Could you check a few things on this model? Use its own coordinates, in mm. Face numbers are marked on the shaded views. A direction names the side the tool comes from. Give positions to 0.01 mm unless a question says otherwise; leave off trailing zeros. Loops run counter-clockwise (first coordinate to the right, second up) from the corner with the lowest first, then second, coordinate; pieces in that order, holes last. Notation, with made-up numbers: (-20.5, -28) -> (-16.5, -28) arc R36 ccw to (-16.5, 7) -> close; hole circle Ø5 at (80, -9). An arc over 180 degrees is marked (long way). Put each result on its own line as item: value.
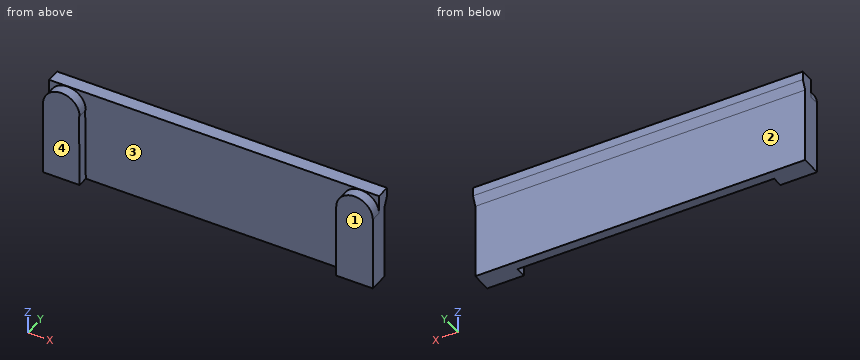
```python
from build123d import *

# Parameters (mm, degrees)
CROQUIS1_W              = 747.21
CROQUIS1_H              = 211.28
SALIENTE_EXTRUIR1_DEPTH = 22
SALIENTE_EXTRUIR6_DEPTH = 39


with BuildPart() as part:
    # Croquis1 → Saliente-Extruir1 (new body)
    with BuildSketch(Plane(origin=(0, 0, 0), x_dir=(1, 0, 0), z_dir=(0, 1, 0))):
        with Locations((318.109210015, -105.64)):
            Rectangle(CROQUIS1_W, CROQUIS1_H)
    extrude(amount=SALIENTE_EXTRUIR1_DEPTH)

    # Croquis2 → Recubrir1 section 0
    with BuildSketch(Plane(origin=(0, 22, 0), x_dir=(1, 0, 0), z_dir=(0, 1, 0))):
        with BuildLine():
            Line((-55.495789985, -171.71895061), (-55.495789985, -211.28))
            Line((-55.495789985, -211.28), (691.714210015, -211.28))
            Line((691.714210015, -211.28), (691.714210015, -171.71895061))
            Line((691.714210015, -171.71895061), (-55.495789985, -171.71895061))
        make_face()
    # Croquis3 → Recubrir1 section 1
    with BuildSketch(Plane(origin=(0, 31, 0), x_dir=(1, 0, 0), z_dir=(0, 1, 0))):
        with BuildLine():
            Line((-55.495789985, -211.28), (-55.495789985, -191.499475305))
            Line((-55.495789985, -191.499475305), (691.714210015, -191.499475305))
            Line((691.714210015, -191.499475305), (691.714210015, -211.28))
            Line((691.714210015, -211.28), (-55.495789985, -211.28))
        make_face()
    loft()

    # Croquis4 → Saliente-Extruir6 (add)
    with BuildSketch(Plane(origin=(0, -24, 0), x_dir=(-1, 0, 0), z_dir=(0, -1, 0))):
        with BuildLine():
            Line((-691.714210015, 0), (-608.79118576, 0))
            Line((-608.79118576, 0), (-608.79118576, -169.061248366))
            ThreePointArc((-608.79118576, -169.061248366), (-650.252697887, -210.522760493), (-691.714210015, -169.061248366))
            Line((-691.714210015, -169.061248366), (-691.714210015, 0))
        make_face()
        with BuildLine():
            Line((55.495789985, 0), (55.495789985, -169.06124837))
            ThreePointArc((55.495789985, -169.06124837), (14.034277855, -210.5227605), (-27.427234275, -169.06124837))
            Line((-27.427234275, -169.06124837), (-26.075334487, -168.034902921))
            Line((-26.075334487, -168.034902921), (-27.427234275, 0))
            Line((-27.427234275, 0), (55.495789985, 0))
        make_face()
    extrude(amount=-SALIENTE_EXTRUIR6_DEPTH)


solid = part.part
```
1. If we section it at A-A (y = -16.5): List the corners of the cut face in (x, z) for me, then the cut area to 3 significant figures.
Recorded:
outline: (-55.5, 0) -> (27.43, 0) -> (26.08, 168.03) -> (27.43, 169.06) arc R41.46 ccw to (-55.5, 169.06) -> close; (608.79, 0) -> (691.71, 0) -> (691.71, 169.06) arc R41.46 ccw to (608.79, 169.06) -> close
area: 33,300 mm^2
2. I'm going to push flat-ended pins straight in: pin 1 (3 mm diameter, centred on x = 213.5, z = 108.5, fed in from -Y); pin 2 (1.5 mm diameter, centred on x = 554, z = 178.5, fed in from +Y); pin 3 (3 mm diameter, centred on x = 581.5, z = 91.5, fed in from +Y). Where does each tip first touch, or does it pass through?
Recorded:
pin 1: stops at y = 0
pin 2: stops at y = 25.43
pin 3: stops at y = 22
3. If we section it at C-C (z = 97): List the corners of the cut face in (x, y) for me, then the cut area to 3 significant figures.
Recorded:
outline: (-55.5, -24) -> (26.65, -24) -> (26.65, 0) -> (608.79, 0) -> (608.79, -24) -> (691.71, -24) -> (691.71, 22) -> (-55.5, 22) -> close
area: 20,400 mm^2
4. Thinking about a two-plate mould opening in X: for the marked faces 3 and 4, which applies, pulls with the +X half, pulls with the -X half, needs draft (parallel to the pull), parting line crosses it, or undercut?
Recorded:
face 3: undercut
face 4: needs draft
5. I need wall thicknesses on line 1 (X direction, y = -12.5, z = 11); line 2 (X direction, y = -3.5, z = 166); line 3 (Y direction, x = 563, z = 80). Which ranges of each line are inside material? Lowest first, please.
Recorded:
line 1: x = -55.5 to 27.34, 608.79 to 691.71
line 2: x = -55.5 to 26.09, 608.79 to 691.71
line 3: y = 0 to 22
6. For the marked faces 1 and 2, which set-ups out of +Z, -Z, +X, -X, +Y, -Y let a thin tool reach every point of the face, with its end or its side?
Recorded:
face 1: +Z, -Z, +X, -X, -Y
face 2: -Z, +X, -X, +Y
7. If we section it at D-D (z = 49.5): List the corners of the cut face in (x, y) for me.
Recorded:
outline: (-55.5, -24) -> (27.03, -24) -> (27.03, 0) -> (608.79, 0) -> (608.79, -24) -> (691.71, -24) -> (691.71, 22) -> (-55.5, 22) -> close
8. If we section it at B-B (x = 143.5): List the corners of the cut face in (y, z) for me.
Recorded:
outline: (0, 0) -> (22, 0) -> (22, 171.72) -> (31, 191.5) -> (31, 211.28) -> (0, 211.28) -> close
